Verification items for the finished model (mm, model axes). A direction names the side the tool comes from. Round coordinates to 2 decimals unless told otherwise and drop trailing zeros. Write each loop counter-clockwise with the first axis right and the second up, starting at its lowest first coordinate (ties: lowest second). Pieces come first, ordered by that corner, then holes. Notation, with made-up numbers: (71, -27) - (127, -27) arc R30 cw to (127, 3) - close; hole circle Ø10 at (1, 51.5). An arc over 180 degrees is marked (long way). Answer as a JSON object with one key per item and string values.
```python
from build123d import *

# Parameters (mm, degrees)
SKETCH_W        = 25.4
SKETCH_H        = 31.75
PAD_DEPTH       = 18.669
POCKET_DEPTH    = 18.67
FILLET_R        = 7.62
POCKET001_DEPTH = 18.67


with BuildPart() as part:
    # Sketch → Pad (new body)
    with BuildSketch(Plane.XY):
        with Locations((12.7, 15.875)):
            Rectangle(SKETCH_W, SKETCH_H)
    extrude(amount=-PAD_DEPTH)

    # Sketch001 (on Face5 of Pad) → Pocket (cut, through all)
    with BuildSketch(Plane.XY):
        Polygon((7.62, 31.75), (0, 30.130319), (0, 31.75), align=None)
    extrude(amount=-POCKET_DEPTH, mode=Mode.SUBTRACT)

    # Fillet
    fillet_edges = [part.edges().sort_by_distance(p)[0] for p in [
        (25.4, 31.75, -9.3345),
        (25.4, 0, -9.3345),
    ]]
    fillet(fillet_edges, radius=FILLET_R)

    # Sketch002 (on Face2 of Fillet) → Pocket001 (cut, through all)
    with BuildSketch(Plane.XY):
        with BuildLine():
            ThreePointArc((12.7, 21.59), (7.62, 16.51), (12.7, 11.43))
            Line((12.7, 11.43), (15.24, 11.43))
            ThreePointArc((15.24, 11.43), (20.32, 16.51), (15.24, 21.59))
            Line((12.7, 21.59), (15.24, 21.59))
        make_face()
    extrude(amount=-POCKET001_DEPTH, mode=Mode.SUBTRACT)


solid = part.part
```
Q1. Section check B-B, the plane z = -3. Record the cut outline in (x, y), then the cut area to 3 significant figures.
Geometry check:
{"outline": "(0, 0) - (17.78, 0) arc R7.62 ccw to (25.4, 7.62) - (25.4, 24.13) arc R7.62 ccw to (17.78, 31.75) - (7.62, 31.75) - (0, 30.13) - close; hole (12.7, 11.43) - (15.24, 11.43) arc R5.08 ccw to (15.24, 21.59) - (12.7, 21.59) arc R5.08 ccw to start", "area": "668 mm2"}
Q2. Section check D-D, the plane y = 28. Record the cut outline in (x, z), then the cut area to 3 significant figures.
Geometry check:
{"outline": "(0, -18.67) - (24.34, -18.67) - (24.34, 0) - (0, 0) - close", "area": "454 mm2"}
Q3. Release check for a two-part mould opening along X. For faces 3 (the flat face through (14, 11.43, -9)), 4 (the flat face through (3.86, 30.95, -9.2)), 5 (the cylindrical face through (23.109, 2.173, -9.465)) record: released by +X, released by -X, zero draft, split by the parting line, or undercut.
Geometry check:
{"face 3": "undercut", "face 4": "released by -X", "face 5": "released by +X"}
Q4. Section check C-C, the plane x = 13.25. Record the cut outline in (y, z), then the cut area to 3 significant figures.
Geometry check:
{"outline": "(0, -18.67) - (11.43, -18.67) - (11.43, 0) - (0, 0) - close; (21.59, -18.67) - (31.75, -18.67) - (31.75, 0) - (21.59, 0) - close", "area": "403 mm2"}
Q5. Section check A-A, the plane y = 16.51. Record the cut outline in (x, z), then the cut area to 3 significant figures.
Geometry check:
{"outline": "(0, -18.67) - (7.62, -18.67) - (7.62, 0) - (0, 0) - close; (20.32, -18.67) - (25.4, -18.67) - (25.4, 0) - (20.32, 0) - close", "area": "237 mm2"}
Q6. Material ranges on line 1 along Y through (x, z) = (17, -13.25); line 2 along Y through (x, z) = (9.75, -13.5); line 3 along X through (y, z) = (16, -6.25), recorded low to high. Write a range as [from, to].
Geometry check:
{"line 1": "y = [0, 11.74], [21.28, 31.75]", "line 2": "y = [0, 12.37], [20.65, 31.75]", "line 3": "x = [0, 7.65], [20.29, 25.4]"}
Q7. Set-up check for faces 1 (the flat face through (14, 21.59, -9)), 2 (the flat face through (25.4, 16, -9)): record each of +Z, -Z, +X, -X, +Y, -Y from which the full face is reachable in a straight line by a thin tool's end or side.
Geometry check:
{"face 1": "+Z, -Z", "face 2": "+Z, -Z, +X, +Y, -Y"}
Q8. Gauge pin test, flat ends, axial feed: P1, Ø1.5, axis at x = 6, y = 27, coming from the +Z side; P2, Ø2, axis at x = 21.5, z = -2, coming from the -Y side. Record the tip position at first contact, or that the pin passes through.
Geometry check:
{"P1": "stops at z = 0", "P2": "stops at y = 0.5"}
